The figure shows three views and two pictorial views of one solid part (mm, origin at its lowest corner). Answer the questions. A direction names the side the tool comes from. Coordinates: 2 decimals unless noted, no trailing zeros. Write each loop counter-clockwise with the first axis right and the second up, starting at its lowest first coordinate (ties: lowest second). Pieces come first, ordered by that corner, then holes. Notation, with made-up numbers: M 3.25,8 L 42.25,8 A26 cw 42.25,28 Z; hole C 79.5,-33.5 d6. An arc over 180 degrees is marked long. Write item = value, one per line.
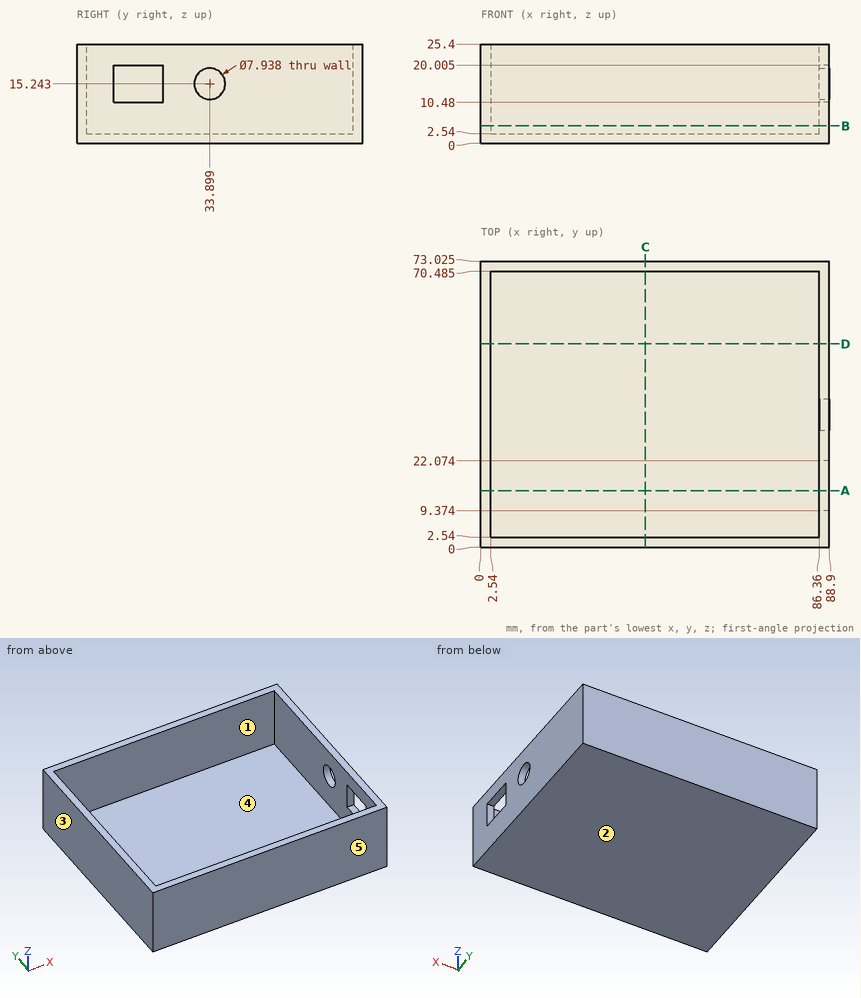
Item 1: Find section C-C (x = 42). Determine the outline of the cut face in (y, z) (1 decimal).
Worked answers:
outline = M 0,0 L 73,0 L 73,25.4 L 70.5,25.4 L 70.5,2.5 L 2.5,2.5 L 2.5,25.4 L 0,25.4 Z
Item 2: Find section A-A (y = 14.5). Determine the outline of the cut face in (x, z) (1 decimal).
Worked answers:
outline = M 0,0 L 88.9,0 L 88.9,10.5 L 86.4,10.5 L 86.4,2.5 L 2.5,2.5 L 2.5,25.4 L 0,25.4 Z; M 86.4,20 L 88.9,20 L 88.9,25.4 L 86.4,25.4 Z
Item 3: Find section D-D (y = 52). Determine the outline of the cut face in (x, z), and give its area (3 significant figures).
Worked answers:
outline = M 0,0 L 88.9,0 L 88.9,25.4 L 86.36,25.4 L 86.36,2.54 L 2.54,2.54 L 2.54,25.4 L 0,25.4 Z
area = 342 mm²
Item 4: Consider line 1 along Y through (x, z) = (48.5, 21) (1 decimal); line 2 along X through (y, z) = (11.5, 23.5); line 3 along Z through (x, y) = (66, 55). Determine where each line is inside the solid, lowest interval first. Write a range as from..to.
Worked answers:
line_1 = 0..2.5, 70.5..73
line_2 = 0..2.54, 86.36..88.9
line_3 = 0..2.54
Item 5: Which of the six approach directions +Z, -Z, +X, -X, +Y, -Y give full straight-line access (tool end or side, diameter ignored) to the marked faces 1 and 2?
Worked answers:
face_1 = +Z
face_2 = -Z, +X, -X, +Y, -Y
Item 6: Find section B-B (z = 4.5). Determine the outline of the cut face in (x, y) (1 decimal).
Worked answers:
outline = M 0,0 L 88.9,0 L 88.9,73 L 0,73 Z; hole M 2.5,2.5 L 86.4,2.5 L 86.4,70.5 L 2.5,70.5 Z
Item 7: For a pull along Y with two mould halves and no side action, classify the marked faces 3, 4 and 5 as released by +Y, released by -Y, zero draft, split by the parting line, or undercut.
Worked answers:
face_3 = zero draft
face_4 = undercut
face_5 = released by -Y
Item 8: Flat-ended cylindrical pins translate along their axes: pin 1 (12 mm diameter, centred on x = 39, y = 43.5, fed in from -Z); pin 2 (8 mm diameter, centred on x = 70.5, y = 57, fed in from +Z). Find the tip coordinate at first contact, or state that the pin passes through.
Worked answers:
pin_1 = 0
pin_2 = 2.54
